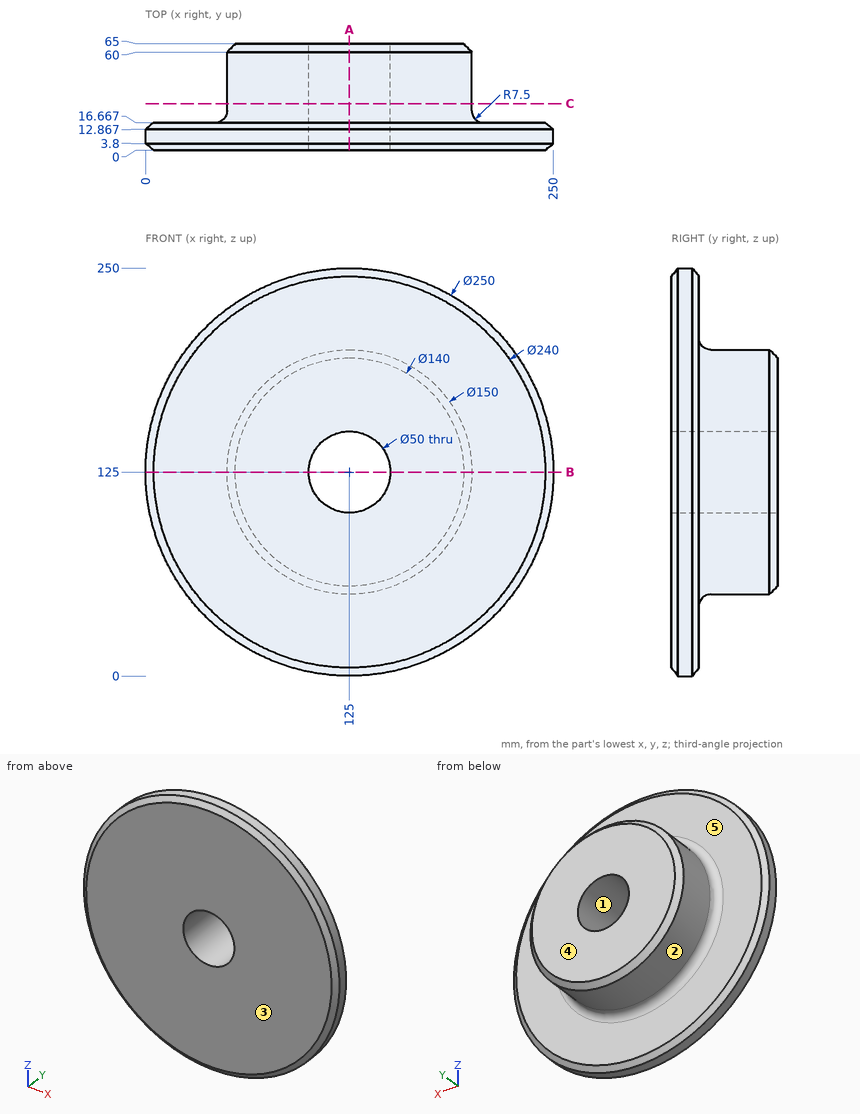
Part print with two shaded views. Sizes in mm from the minimum x, y, z corner. A direction names the side the tool comes from. Coordinates: 2 decimals unless noted, no trailing zeros. Order: outer loops, then holes, each group sorted by start corner. A loop starts at its lowest first (then second) coordinate and runs counter-clockwise, first axis right, second up.
(1) Saw through at C-C, the plane y = 28.5. Write the cut outline in (x, z).
Solution:
outline: circle Ø150 at (125, 125); hole circle Ø50 at (125, 125)
(2) Saw through at A-A, the plane x = 125. Write the cut outline in (y, z), and give its area (3 significant figures).
Solution:
outline: (0, 5) - (3.8, 0) - (12.87, 0) - (16.67, 5) - (16.67, 42.5) arc R7.5 cw to (24.17, 50) - (60, 50) - (65, 55) - (65, 100) - (0, 100) - close; (0, 150) - (65, 150) - (65, 195) - (60, 200) - (24.17, 200) arc R7.5 cw to (16.67, 207.5) - (16.67, 245) - (12.87, 250) - (3.8, 250) - (0, 245) - close
area: 8,130 mm2
(3) Mould opens along Z. For the marked faces 1, 2 and 3 say: released by +Z, released by -Z, zero draft, split by the parting line, or undercut.
Solution:
face 1: undercut
face 2: split by the parting line
face 3: zero draft
(4) Drill centre lines: L1, parallel to X at y = 38, z = 125; L2, parallel to X at y = 20, z = 125 (1 decimal); L3, parallel to Y at x = 132.5, z = 11. Where is each one in solid material? Low to high.
Solution:
L1: x = 50 to 100, 150 to 200
L2: x = 48.7 to 100, 150 to 201.3
L3: y = 0 to 16.67
(5) Saw through at B-B, the plane z = 125. Write the cut outline in (x, y), and give its area (3 significant figures).
Solution:
outline: (0, 3.8) - (5, 0) - (100, 0) - (100, 65) - (55, 65) - (50, 60) - (50, 24.17) arc R7.5 cw to (42.5, 16.67) - (5, 16.67) - (0, 12.87) - close; (150, 0) - (245, 0) - (250, 3.8) - (250, 12.87) - (245, 16.67) - (207.5, 16.67) arc R7.5 cw to (200, 24.17) - (200, 60) - (195, 65) - (150, 65) - close
area: 8,130 mm2
(6) Which spindle directions (+Z, -Z, +X, -X, +Y, -Y) get a long thin tool onto all of the face, cutting with end or side? Do the marked faces 4 and 5. Say none if no direction does.
Solution:
face 4: +Z, -Z, +X, -X, +Y
face 5: +Y
(7) Pin check, flat tips, straight feed: pin 1 Ø6 at (y, z) = (15.5, 54) entering from -X (1 decimal); pin 2 Ø4 at (y, z) = (36.5, 59) entering from +X; pin 3 Ø6 at (x, y) = (223, 7) entering from -Z; pin 4 Ø1.5 at (x, z) = (215, 118.5) entering from -Y. Stop position of each tip, or through.
Solution:
pin 1: stops at x = 21.1
pin 2: stops at x = 164.1
pin 3: stops at z = 43.76
pin 4: stops at y = 0
